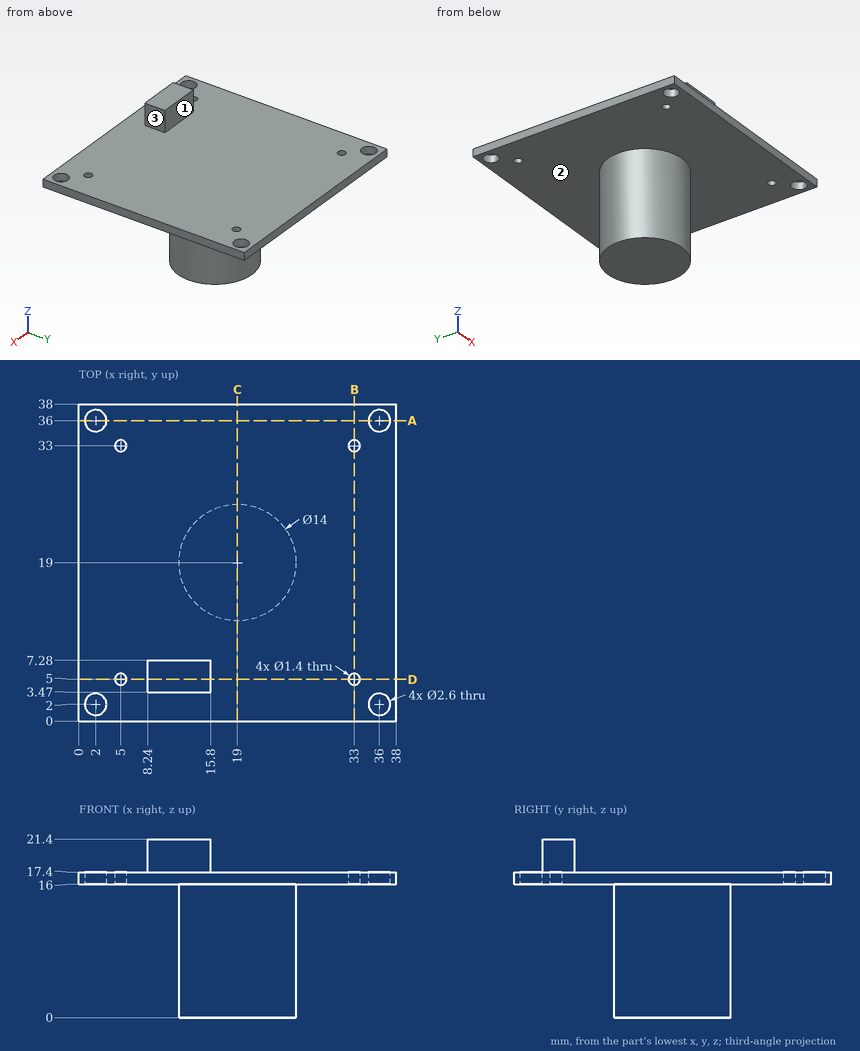
Geometry: see drawing. Coordinates: mm, zero at the bounding-box minimum. A direction names the side the tool comes from. Coordinates: 2 decimals unless noted, no trailing zeros. Loops run counter-clockwise (first coordinate to the right, second up) from the corner with the lowest first, then second, coordinate; pieces in that order, holes last. Notation, with made-up numbers: (19, -9) - (37, -9) arc R14 cw to (37, 13) - close; hole circle Ø4 at (21.5, -3.5). An arc over 180 degrees is marked (long way). Put each result on its own line as item: value. Start each with the question number.
Q1. Line query: line 1 (X direction, y = 33, z = 16.4); line 2 (Y direction, x = 36, z = 16.6). Output: solid intervals per line, ascending.
Q2. Cut plane C-C, the plane x = 19. Return loops of the section in (y, z), and give its area (3 significant figures).
Q3. Cut plane D-D, the plane y = 5. Return loops of the section in (x, z).
Q4. Cut plane B-B, the plane x = 33. Return loops of the section in (y, z), and give its area (3 significant figures).
Q5. Set-up query: the marked faces 1, 2 and 3. Return all of +Z, -Z, +X, -X, +Y, -Y with unobstructed straight access to the full face (end or side cutting, diameter ignored); none if empty.
Q6. Pin query (flat end, axial travel): pin 1 Ø2.5 at (x, y) = (36, 2) entering from +Z; pin 2 Ø1.5 at (x, z) = (20.5, 2.5) entering from -Y; pin 3 Ø3.5 at (x, y) = (2, 36) entering from +Z; pin 4 Ø10 at (y, z) = (18.5, 6) entering from -X. Return the tip coordinate at first contact, or that it passes through.
Q7. Cut plane A-A, the plane y = 36. Return loops of the section in (x, z).
Filled sheet:
1. line 1: 0 to 4.3, 5.7 to 32.3, 33.7 to 38
1. line 2: 0 to 0.7, 3.3 to 34.7, 37.3 to 38
2. outline: (0, 16) - (12, 16) - (12, 0) - (26, 0) - (26, 16) - (38, 16) - (38, 17.4) - (0, 17.4) - close
2. area: 277 mm²
3. outline: (0, 16) - (4.3, 16) - (4.3, 17.4) - (0, 17.4) - close; (5.7, 16) - (32.3, 16) - (32.3, 17.4) - (15.8, 17.4) - (15.8, 21.4) - (8.24, 21.4) - (8.24, 17.4) - (5.7, 17.4) - close; (33.7, 16) - (38, 16) - (38, 17.4) - (33.7, 17.4) - close
4. outline: (0, 16) - (4.3, 16) - (4.3, 17.4) - (0, 17.4) - close; (5.7, 16) - (32.3, 16) - (32.3, 17.4) - (5.7, 17.4) - close; (33.7, 16) - (38, 16) - (38, 17.4) - (33.7, 17.4) - close
4. area: 49.3 mm²
5. face 1: +Z, +X, -X, +Y
5. face 2: -Z
5. face 3: +Z, +X, +Y, -Y
6. pin 1: through
6. pin 2: y = 12.04
6. pin 3: z = 17.4
6. pin 4: x = 12
7. outline: (0, 16) - (0.7, 16) - (0.7, 17.4) - (0, 17.4) - close; (3.3, 16) - (34.7, 16) - (34.7, 17.4) - (3.3, 17.4) - close; (37.3, 16) - (38, 16) - (38, 17.4) - (37.3, 17.4) - close
